Geometry check sheet. Reference: the model listing, model coordinates, mm. Face numbers are marked on the shaded views. Round coordinates to 2 decimals unless told otherwise and drop trailing zeros. Order: outer loops, then holes, each group sorted by start corner. A loop starts at its lowest first (then second) coordinate and runs counter-clockwise, first axis right, second up. Notation, with made-up numbers: M -20.5,75 L -7.5,75 A24 cw -7.5,94 Z; hole C 6.5,48.5 d8. An arc over 180 degrees is marked long. Answer as a JSON object with one key per item and string values. Group by question number.
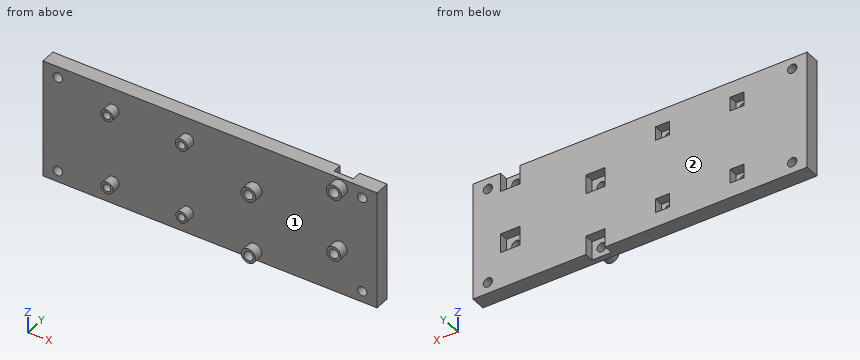
```python
from build123d import *

# Parameters (mm, degrees)
SKETCH1_W           = 114.3
SKETCH1_H           = 40.64
BOSS_EXTRUDE1_DEPTH = 5.08
SKETCH2_R           = 1.5875
CUT_EXTRUDE1_DEPTH  = 84.991521289
SKETCH5_R           = 1.5875
CUT_EXTRUDE2_DEPTH  = 84.991521289
BOSS_EXTRUDE2_START = 3.175
SKETCH6_R           = 2.575286713
SKETCH6_R_2         = 1.755660025
SKETCH6_R_3         = 2.467274827
SKETCH6_R_4         = 1.5875
SKETCH6_R_5         = 2.529262395
SKETCH6_R_6         = 2.491560895
BOSS_EXTRUDE2_DEPTH = 3.175
SKETCH7_R           = 1.27
CUT_EXTRUDE3_DEPTH  = 84.991521289
BOSS_EXTRUDE3_START = 3.175
SKETCH8_R           = 2.037414518
SKETCH8_R_2         = 1.27
SKETCH8_R_3         = 2.098900923
SKETCH8_R_4         = 1.95707153
SKETCH8_R_5         = 2.085151837
BOSS_EXTRUDE3_DEPTH = 3.175
SKETCH9_W           = 6.604
SKETCH9_H           = 6.604
SKETCH9_W_2         = 4.826
SKETCH9_H_2         = 4.826
CUT_EXTRUDE4_DEPTH  = 3.175


with BuildPart() as part:
    # Sketch1 → Boss-Extrude1 (new body)
    with BuildSketch(Plane(origin=(0, 0, 0), x_dir=(1, 0, 0), z_dir=(0, 1, 0))):
        with Locations((19.44536493, 13.766937669)):
            Rectangle(SKETCH1_W, SKETCH1_H)
    extrude(amount=BOSS_EXTRUDE1_DEPTH)

    # Sketch2 → Cut-Extrude1 (cut, through all)
    with BuildSketch(Plane(origin=(0, 5.08, 0), x_dir=(1, 0, 0), z_dir=(0, 1, 0))):
        with Locations(Location((-32.62463507, 30.276937669, 0), (0, 0, 270))):
            Circle(SKETCH2_R)
        with Locations(Location((71.51536493, 30.276937669, 0), (0, 0, 270))):
            Circle(SKETCH2_R)
        with Locations(Location((71.51536493, -2.743062331, 0), (0, 0, 270))):
            Circle(SKETCH2_R)
        with Locations(Location((-32.62463507, -2.743062331, 0), (0, 0, 270))):
            Circle(SKETCH2_R)
    extrude(amount=-CUT_EXTRUDE1_DEPTH, mode=Mode.SUBTRACT)

    # Sketch5 → Cut-Extrude2 (cut, through all)
    with BuildSketch(Plane.XZ):
        with Locations(Location((63.89536493, 3.378062331, 0), (0, 0, 270))):
            Circle(SKETCH5_R)
        with Locations(Location((34.68536493, -9.321937669, 0), (0, 0, 270))):
            Circle(SKETCH5_R)
        with Locations(Location((63.89536493, -18.211937669, 0), (0, 0, 270))):
            Circle(SKETCH5_R)
        with Locations(Location((34.68536493, -30.911937669, 0), (0, 0, 270))):
            Circle(SKETCH5_R)
    extrude(amount=-CUT_EXTRUDE2_DEPTH, mode=Mode.SUBTRACT)

    # Sketch6 → Boss-Extrude2 (add)
    # profile 1 of 4: a face of its own
    with BuildSketch(Plane.XZ.offset(BOSS_EXTRUDE2_START)):
        with Locations(Location((63.89536493, 3.378062331, 0), (0, 0, 270))):
            Circle(SKETCH6_R)
        with Locations(Location((63.89536493, 3.378062331, 0), (0, 0, 270))):
            Circle(SKETCH6_R_2, mode=Mode.SUBTRACT)
    # profile 2 of 4: a face of its own
    with BuildSketch(Plane.XZ.offset(BOSS_EXTRUDE2_START)):
        with Locations(Location((63.89536493, -18.211937669, 0), (0, 0, 270))):
            Circle(SKETCH6_R_3)
        with Locations(Location((63.89536493, -18.211937669, 0), (0, 0, 270))):
            Circle(SKETCH6_R_4, mode=Mode.SUBTRACT)
    # profile 3 of 4: a face of its own
    with BuildSketch(Plane.XZ.offset(BOSS_EXTRUDE2_START)):
        with Locations(Location((34.68536493, -9.321937669, 0), (0, 0, 270))):
            Circle(SKETCH6_R_5)
        with Locations(Location((34.68536493, -9.321937669, 0), (0, 0, 270))):
            Circle(SKETCH6_R_4, mode=Mode.SUBTRACT)
    # profile 4 of 4: a face of its own
    with BuildSketch(Plane.XZ.offset(BOSS_EXTRUDE2_START)):
        with Locations(Location((34.68536493, -30.911937669, 0), (0, 0, 270))):
            Circle(SKETCH6_R_6)
        with Locations(Location((34.68536493, -30.911937669, 0), (0, 0, 270))):
            Circle(SKETCH6_R_4, mode=Mode.SUBTRACT)
    extrude(amount=-BOSS_EXTRUDE2_DEPTH)

    # Sketch7 → Cut-Extrude3 (cut, through all)
    with BuildSketch(Plane.XZ):
        with Locations(Location((11.764327972, -1.084047056, 0), (0, 0, 270))):
            Circle(SKETCH7_R)
        with Locations(Location((11.771660973, -26.584045801, 0), (0, 0, 270))):
            Circle(SKETCH7_R)
        with Locations(Location((-13.735671828, -1.084047056, 0), (0, 0, 270))):
            Circle(SKETCH7_R)
        with Locations(Location((-13.728338827, -26.584045801, 0), (0, 0, 270))):
            Circle(SKETCH7_R)
    extrude(amount=-CUT_EXTRUDE3_DEPTH, mode=Mode.SUBTRACT)

    # Sketch8 → Boss-Extrude3 (add)
    # profile 1 of 4: a face of its own
    with BuildSketch(Plane.XZ.offset(BOSS_EXTRUDE3_START)):
        with Locations(Location((-13.735671828, -1.084047056, 0), (0, 0, 270))):
            Circle(SKETCH8_R)
        with Locations(Location((-13.735671828, -1.084047056, 0), (0, 0, 270))):
            Circle(SKETCH8_R_2, mode=Mode.SUBTRACT)
    # profile 2 of 4: a face of its own
    with BuildSketch(Plane.XZ.offset(BOSS_EXTRUDE3_START)):
        with Locations(Location((11.764327972, -1.084047056, 0), (0, 0, 270))):
            Circle(SKETCH8_R_3)
        with Locations(Location((11.764327972, -1.084047056, 0), (0, 0, 270))):
            Circle(SKETCH8_R_2, mode=Mode.SUBTRACT)
    # profile 3 of 4: a face of its own
    with BuildSketch(Plane.XZ.offset(BOSS_EXTRUDE3_START)):
        with Locations(Location((11.771660973, -26.584045801, 0), (0, 0, 270))):
            Circle(SKETCH8_R_4)
        with Locations(Location((11.771660973, -26.584045801, 0), (0, 0, 270))):
            Circle(SKETCH8_R_2, mode=Mode.SUBTRACT)
    # profile 4 of 4: a face of its own
    with BuildSketch(Plane.XZ.offset(BOSS_EXTRUDE3_START)):
        with Locations(Location((-13.728338827, -26.584045801, 0), (0, 0, 270))):
            Circle(SKETCH8_R_5)
        with Locations(Location((-13.728338827, -26.584045801, 0), (0, 0, 270))):
            Circle(SKETCH8_R_2, mode=Mode.SUBTRACT)
    extrude(amount=-BOSS_EXTRUDE3_DEPTH)

    # Sketch9 → Cut-Extrude4 (cut)
    with BuildSketch(Plane(origin=(0, 5.08, 0), x_dir=(1, 0, 0), z_dir=(0, 1, 0))):
        with Locations((63.89536493, 18.211937669)):
            Rectangle(SKETCH9_W, SKETCH9_H)
        with Locations((63.89536493, -3.378062331)):
            Rectangle(SKETCH9_W, SKETCH9_H)
        with Locations((34.68536493, 9.321937669)):
            Rectangle(SKETCH9_W, SKETCH9_H)
        with Locations((34.68536493, 30.911937669)):
            Rectangle(SKETCH9_W, SKETCH9_H)
        with Locations((-13.728338827, 26.584045801)):
            Rectangle(SKETCH9_W_2, SKETCH9_H_2)
        with Locations((11.771660973, 26.584045801)):
            Rectangle(SKETCH9_W_2, SKETCH9_H_2)
        with Locations((-13.735671828, 1.084047056)):
            Rectangle(SKETCH9_W_2, SKETCH9_H_2)
        with Locations((11.764327972, 1.084047056)):
            Rectangle(SKETCH9_W_2, SKETCH9_H_2)
    extrude(amount=-CUT_EXTRUDE4_DEPTH, mode=Mode.SUBTRACT)


solid = part.part
```
1) Go/stop test with flat-tipped pins: P1, Ø1.4, axis at x = -14.5, z = -1.5, coming from the +Y side (3 decimals); P2, Ø8, axis at x = 0, z = -15, coming from the -Y side; P3, Ø1.6, axis at x = 33, y = 4, coming from the -Z side. Record where each tip stops, or that it passes through.
2) Sectioned sample at B-B (z = -18). Record the boundary of the cut face in (x, y) (3 decimals), then the cut area to 3 significant figures.
3) Sectioned sample at D-D (z = -5). Record the boundary of the cut face in (x, y).
4) Thickness scan on line 1 along X through (y, z) = (4.25, -2); line 2 along Z through (x, y) = (-16, 4); line 3 along X through (y, z) = (3, -20). Record the ranges inside material, lowest first. Write a range as [from, to].
5) Release check for a two-part mould opening along Y. For the marked faces 1 and 2 record: +Y half, -Y half, draft (parallel to the pull), parting line (faces both ways), or undercut.
6) Sectioned sample at A-A (y = -1). Count the separate pieces of the cut face and the enclosed holes in it, then the cut area to 3 significant figures.
7) Sectioned sample at C-C (x = 19.5). Record the boundary of the cut face in (y, z).
Final values:
{
 "1": {"P1": "stops at y = 1.905", "P2": "stops at y = 0", "P3": "stops at z = -27.61"},
 "2": {"outline": "M -37.705,0 L 61.437,0 L 61.437,-3.175 L 62.322,-3.175 L 62.322,1.905 L 60.593,1.905 L 60.593,5.08 L -37.705,5.08 Z; M 65.469,-3.175 L 66.354,-3.175 L 66.354,0 L 76.595,0 L 76.595,5.08 L 67.197,5.08 L 67.197,1.905 L 65.469,1.905 Z", "area": "559 mm^2"},
 "3": {"outline": "M -37.7,0 L 76.6,0 L 76.6,5.08 L -37.7,5.08 Z"},
 "4": {"line 1": "x = [-37.7, -16.15], [-11.32, 9.35], [14.18, 76.6]", "line 2": "z = [-34.09, -29], [-24.17, -3.5], [1.33, 6.55]", "line 3": "x = [-37.7, 60.59], [67.2, 76.6]"},
 "5": {"face 1": "-Y half", "face 2": "+Y half"},
 "6": {"separate pieces": "8", "enclosed holes": "8", "area": "78.4 mm^2"},
 "7": {"outline": "M 0,-34.09 L 5.08,-34.09 L 5.08,6.55 L 0,6.55 Z"}
}
